Model file for the job. Use its own axes, mm. A direction names the side the tool comes from. Give positions to 0.01 mm unless a question says otherwise; leave off trailing zeros. Loops run counter-clockwise (first coordinate to the right, second up) from the corner with the lowest first, then second, coordinate; pieces in that order, holes last. Notation, with made-up numbers: (32, 17) - (71, 17) arc R14 cw to (71, 40) - close; hole circle Ø1 at (-3.5, 76.5). An arc over 180 degrees is marked (long way). Use a Markdown table: item, result.
from build123d import *

# Parameters (mm, degrees)
BOSS_EXTRUDE1_DEPTH = 180
SKETCH2_R           = 2.75
CUT_EXTRUDE1_DEPTH  = 1


with BuildPart() as part:
    # Sketch1 → Boss-Extrude1 (new body)
    with BuildSketch(Plane.XY):
        with BuildLine():
            Line((2, 0), (25, 0))
            ThreePointArc((25, 0), (26.414213562, 0.585786438), (27, 2))
            Line((27, 2), (27, 5.5))
            ThreePointArc((27, 5.5), (27.292893219, 6.207106781), (28, 6.5))
            Line((28, 6.5), (31, 6.5))
            Line((31, 6.5), (31, 7.5))
            Line((31, 7.5), (28, 7.5))
            ThreePointArc((28, 7.5), (26.585786438, 6.914213562), (26, 5.5))
            Line((26, 5.5), (26, 2))
            ThreePointArc((26, 2), (25.707106781, 1.292893219), (25, 1))
            Line((25, 1), (2, 1))
            ThreePointArc((2, 1), (1.292893219, 1.292893219), (1, 2))
            Line((1, 2), (1, 4.544540718))
            ThreePointArc((1, 4.544540718), (0.414213562, 5.95875428), (-1, 6.544540718))
            Line((-1, 6.544540718), (-4, 6.544540718))
            Line((-4, 6.544540718), (-4, 5.544540718))
            Line((-4, 5.544540718), (-1, 5.544540718))
            ThreePointArc((-1, 5.544540718), (-0.292893219, 5.251647499), (0, 4.544540718))
            Line((0, 4.544540718), (0, 2))
            ThreePointArc((0, 2), (0.585786438, 0.585786438), (2, 0))
        make_face()
    extrude(amount=BOSS_EXTRUDE1_DEPTH)

    # Sketch2 → Cut-Extrude1 (cut)
    with BuildSketch(Plane(origin=(0, 1, 0), x_dir=(1, 0, 0), z_dir=(0, 1, 0))):
        with Locations(Location((13.5, -10, 0), (0, 0, 270))):
            Circle(SKETCH2_R)
        with Locations(Location((13.5, -170, 0), (0, 0, 270))):
            Circle(SKETCH2_R)
    extrude(amount=-CUT_EXTRUDE1_DEPTH, mode=Mode.SUBTRACT)


solid = part.part
(1) Slice it at B-B, the plane z = 10. Write the cut outline in (x, y).
Computed:
| item | result |
|---|---|
| outline | (-4, 5.54) - (-1, 5.54) arc R1 cw to (0, 4.54) - (0, 2) arc R2 ccw to (2, 0) - (10.75, 0) - (10.75, 1) - (2, 1) arc R1 cw to (1, 2) - (1, 4.54) arc R2 ccw to (-1, 6.54) - (-4, 6.54) - close; (16.25, 0) - (25, 0) arc R2 ccw to (27, 2) - (27, 5.5) arc R1 cw to (28, 6.5) - (31, 6.5) - (31, 7.5) - (28, 7.5) arc R2 ccw to (26, 5.5) - (26, 2) arc R1 cw to (25, 1) - (16.25, 1) - close |
(2) Slice it at D-D, the plane z = 82. Write the cut outline in (x, y), plus the area to 3 significant figures.
Computed:
| item | result |
|---|---|
| outline | (-4, 5.54) - (-1, 5.54) arc R1 cw to (0, 4.54) - (0, 2) arc R2 ccw to (2, 0) - (25, 0) arc R2 ccw to (27, 2) - (27, 5.5) arc R1 cw to (28, 6.5) - (31, 6.5) - (31, 7.5) - (28, 7.5) arc R2 ccw to (26, 5.5) - (26, 2) arc R1 cw to (25, 1) - (2, 1) arc R1 cw to (1, 2) - (1, 4.54) arc R2 ccw to (-1, 6.54) - (-4, 6.54) - close |
| area | 44.5 mm² |
(3) Pin check, flat tips, straight feed: P1, Ø3.5, axis at x = -3, z = 78.5, coming from the -Y side; P2, Ø1, axis at y = 1, z = 71.5, coming from the +X side; P3, Ø1, axis at y = 3, z = 110, coming from the +X side; P4, Ø5, axis at x = 13.5, z = 170, coming from the +Y side. Stop position of each tip, or through.
Computed:
| item | result |
|---|---|
| P1 | y = 5.54 |
| P2 | x = 26.94 |
| P3 | x = 27 |
| P4 | through |
(4) Drill centre lines: probe 1 along X at (y, z) = (2.25, 85); probe 2 along Y at (x, z) = (24.5, 170.5); probe 3 along Y at (x, z) = (-2, 138.5). Where is each one in solid material? Low to high. Write a range as [from, to].
Computed:
| item | result |
|---|---|
| probe 1 | [0, 1], [26, 27] |
| probe 2 | [0, 1] |
| probe 3 | [5.54, 6.54] |
(5) 3-axis set-ups, long thin cutter, end or side, ignore diameter. For faces 1 (the flat face through (26, 4, 89)), 2 (the flat face through (-3, 5.545, 89)), 3 (the flat face through (13.4, 0.7, 180)), 4 (the flat face through (-2, 6.545, 89)), 5 (the flat face through (13, 0, 89)): which of +Z, -Z, +X, -X, +Y, -Y reach the whole face in a straight line?
Computed:
| item | result |
|---|---|
| face 1 | +Z, -Z, +Y |
| face 2 | +Z, -Z, -X, -Y |
| face 3 | +Z, +X, -X, +Y, -Y |
| face 4 | +Z, -Z, -X, +Y |
| face 5 | +Z, -Z, +X, -X, -Y |
(6) Mould opens along Y. For faces 6 (the flat face through (30, 7.5, 89)), 7 (the flat face through (27, 4, 89)), 8 (the flat face through (29, 6.5, 89)) say: pulls with the +Y half, pulls with the -Y half, needs draft (parallel to the pull), parting line crosses it, or undercut.
Computed:
| item | result |
|---|---|
| face 6 | pulls with the +Y half |
| face 7 | needs draft |
| face 8 | pulls with the -Y half |
(7) Slice it at A-A, the plane y = 3.25. Write the cut outline in (x, z).
Computed:
| item | result |
|---|---|
| outline | (0, 0) - (1, 0) - (1, 180) - (0, 180) - close; (26, 0) - (27, 0) - (27, 180) - (26, 180) - close |
(8) Slice it at C-C, the plane x = 13.5. Write the cut outline in (y, z).
Computed:
| item | result |
|---|---|
| outline | (0, 0) - (1, 0) - (1, 7.25) - (0, 7.25) - close; (0, 12.75) - (1, 12.75) - (1, 167.25) - (0, 167.25) - close; (0, 172.75) - (1, 172.75) - (1, 180) - (0, 180) - close |
